from build123d import *

# Parameters (mm, degrees)
F2_R           = 1.5875
F3_DEPTH       = 25.4
F6_DEPTH       = 2.54
F8_W           = 5.08
F8_H           = 12.7
F9_DEPTH       = 17.3480194062
F10_W          = 3.175
F10_H          = 3.175
F11_DEPTH      = 7.62
F12_R          = 0.396875
F13_DEPTH      = 25.4
F13_DEPTH_BACK = 25.4
F14_R          = 0.3175
F15_DEPTH      = 0.635
F16_R          = 0.635
F17_DEPTH      = 8.2660857588
F18_W          = 2.54
F18_H          = 3.8718514089
F19_DEPTH      = 25.4
F20_SIZE       = 0.508


with BuildPart() as f1:
    # F0 (on Right) → F1 (revolve)
    with BuildSketch(Plane.YZ):
        Polygon((26.67, 3.175), (26.67, 0), (50.8, 0), (50.8, 3.81), (31.75, 3.81), (31.75, 6.35), (0, 6.35), (0, 5.08), (1.143, 5.08), (1.143, 0.3175), (2.286, 0.3175), (2.286, 3.175), align=None)
    revolve(axis=Axis((0, 38.735, 0), (0, 1, 0)))

    # F2 (on Right) → F3 (cut)
    with BuildSketch(Plane.YZ):
        with Locations((40.64, 0)):
            Circle(F2_R)
    extrude(amount=F3_DEPTH, mode=Mode.SUBTRACT)

    # F5 (on offset) → F6 (cut)
    with BuildSketch(Plane.YZ.offset(-6.35)):
        with BuildLine():
            Line((4.7625, -1.5875), (23.8125, -1.5875))
            ThreePointArc((23.8125, -1.5875), (25.4, 0), (23.8125, 1.5875))
            Line((23.8125, 1.5875), (4.7625, 1.5875))
            ThreePointArc((4.7625, 1.5875), (3.175, 0), (4.7625, -1.5875))
        make_face()
    extrude(amount=F6_DEPTH, mode=Mode.SUBTRACT)

    # F8 (on offset) → F9 (cut)
    with BuildSketch(Plane.XZ.offset(-13.112607412)):
        with Locations((0, -7.6607518819)):
            Rectangle(F8_W, F8_H)
    extrude(amount=-F9_DEPTH, mode=Mode.SUBTRACT)

    # F10 (on face) → F11 (cut)
    with BuildSketch(Plane.XZ):
        with Locations((0, 6.0977916799)):
            Rectangle(F10_W, F10_H)
    extrude(amount=-F11_DEPTH, mode=Mode.SUBTRACT)

    # F12 (on face) → F13 (cut, two sides)
    with BuildSketch(Plane(origin=(1.5875, 0, 0), x_dir=(0, -1, 0), z_dir=(-1, 0, 0))) as f13_sk:
        with Locations((-4.3815, 5.2224572188)):
            Circle(F12_R)
    extrude(amount=-F13_DEPTH, mode=Mode.SUBTRACT)
    extrude(f13_sk.sketch, amount=F13_DEPTH_BACK, mode=Mode.SUBTRACT)

    # F14 (on face) → F15 (cut)
    with BuildSketch(Plane.XY.offset(4.5102916799)):
        with Locations((0, 6.35)):
            Circle(F14_R)
    extrude(amount=-F15_DEPTH, mode=Mode.SUBTRACT)

    # F16 (on face) → F17 (cut)
    with BuildSketch(Plane(origin=(0, 31.75, 0), x_dir=(-1, 0, 0), z_dir=(0, 1, 0))):
        with Locations((0, 5.08)):
            Circle(F16_R)
    extrude(amount=-F17_DEPTH, mode=Mode.SUBTRACT)

    # F18 (on face) → F19 (cut)
    with BuildSketch(Plane.XZ):
        with Locations((0, -6.3809257044)):
            Rectangle(F18_W, F18_H)
    extrude(amount=-F19_DEPTH, mode=Mode.SUBTRACT)

    # F20
    f20_edges = [f1.edges().sort_by_distance(p)[0] for p in [
        (0, 50.8, -3.81),
    ]]
    chamfer(f20_edges, length=F20_SIZE)


solid = f1.part
Read the model definition and answer for the solid it produces. Units are mm, in the model's axes. A direction names the side the tool comes from. Coordinates: 2 decimals unless noted, no trailing zeros. Loops run counter-clockwise (first coordinate to the right, second up) from the corner with the lowest first, then second, coordinate; pieces in that order, holes last.
Q1. Which of the six approach directions +Z, -Z, +X, -X, +Y, -Y give full straight-line access (tool end or side, diameter ignored) to faces 1 (the face through (-5, 14, 1.588)), 2 (the face through (0, 7.62, 5)), 3 (the face through (0, 7, -4.445)), 4 (the face through (0, 1.143, 1)), 5 (the face through (2.54, 22, -4))?
Q2. The part is cut by section A-A on y = 28. Write down the section's boundary in (x, z) (3 decimals).
Q3. Consider probe 1 along Y at (x, z) = (2.2, 0); probe 2 along X at (y, z) = (13.5, -0.25); probe 3 along Y at (x, z) = (-2, -5.5). Determine where each line is inside the solid, lowest interval first.
Q4. The part is cut by section B-B on y = 40.64. Write down the section's boundary in (x, z), and give its area (3 significant figures).
Q5. The mould has two halves that part along Z. Classify faces 6 (the face through (0, 41, 0)), 7 (the face through (-0.293, 27.675, 4.517)), 8 (the face through (0, 50.8, 0)), 9 (the face through (0, 29, -1.311)): +Z half, -Z half, draft (parallel to the pull), parting line (faces both ways), or undercut.
Q6. Each of these flat-tipped pins is pushed along its axis until it touches: pin 1 Ø4 at (x, z) = (0.5, 0) entering from -Y; pin 2 Ø5 at (y, z) = (17.5, -4.5) entering from -X; pin 3 Ø3.5 at (y, z) = (40.64, 0) entering from -X. Where does it stop, or does it pass through?
Results below:
1. face 1: -X
1. face 2: +Z, -Y
1. face 3: -Z, -Y
1. face 4: -Y
1. face 5: -Z
2. outline: (-2.54, -5.82) - (-2.54, -1.311) - (2.54, -1.311) - (2.54, -5.82) arc R6.35 ccw (long way) to start; hole circle Ø1.27 at (0, 5.08)
3. probe 1: y = 1.14 to 2.29, 26.67 to 39.05, 42.23 to 50.8
3. probe 2: x = -3.81 to -3.17, 3.17 to 6.35
3. probe 3: y = 0 to 13.11, 30.46 to 31.75
4. outline: (0, -1.59) - (0, 1.59) - (3.46, 1.59) arc R3.81 ccw (long way) to (3.46, -1.59) - close
4. area: 33.9 mm2
5. face 6: undercut
5. face 7: undercut
5. face 8: draft
5. face 9: -Z half
6. pin 1: stops at y = 1.14
6. pin 2: stops at x = -6.03
6. pin 3: stops at x = -3.81
